The model under review builds one solid part; all positions refer to its coordinate system, in mm. Face numbers are marked on the shaded views. A direction names the side the tool comes from. Coordinates: 2 decimals unless noted, no trailing zeros. Loops run counter-clockwise (first coordinate to the right, second up) from the corner with the lowest first, then second, coordinate; pieces in that order, holes last. Notation, with made-up numbers: M 10.25,39.25 L 37.25,39.25 A19 cw 37.25,61.25 Z; hole C 35.25,-1.75 d10. An arc over 180 degrees is marked long. One line per item, written item: value.
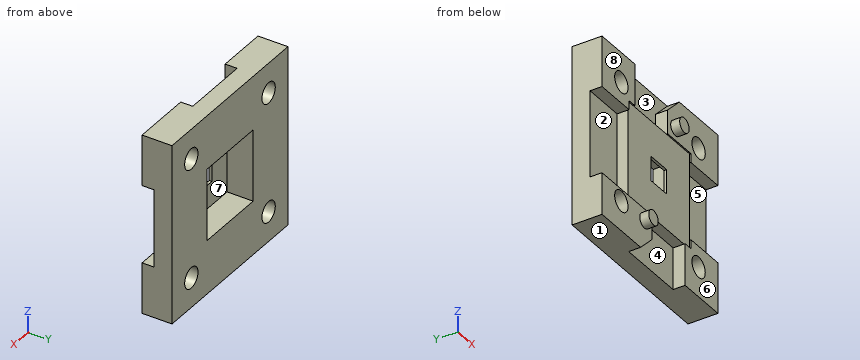
```python
from build123d import *

# Parameters (mm, degrees)
SKETCH_W        = 30
SKETCH_H        = 30
PAD_DEPTH       = 5
SKETCH001_W     = 7
SKETCH001_H     = 23
SKETCH001_W_2   = 23
SKETCH001_H_2   = 7
SKETCH001_H_3   = 16
SKETCH001_W_3   = 30
POCKET_DEPTH    = 2
SKETCH002_W     = 13
SKETCH002_H     = 7
PAD001_DEPTH    = 2
SKETCH003_R     = 1.725
POCKET001_DEPTH = 5.001
SKETCH004_R     = 1.225
PAD002_DEPTH    = 1.5
SKETCH005_W     = 7
SKETCH005_H     = 2
PAD003_DEPTH    = 1.5
SKETCH006_W     = 4.1
SKETCH006_H     = 4.1
POCKET002_DEPTH = 5
PAD004_DEPTH    = 2
SKETCH008_R     = 1.725
POCKET003_DEPTH = 5.001
PAD005_DEPTH    = 2
SKETCH010_R     = 1.725
POCKET004_DEPTH = 5.001
POCKET005_DEPTH = 2
SKETCH012_W     = 13
SKETCH012_H     = 7
PAD006_DEPTH    = 2
SKETCH013_R     = 1.725
POCKET006_DEPTH = 5.001
SKETCH014_R     = 1.225
PAD007_DEPTH    = 1.5
POCKET007_DEPTH = 2
SKETCH016_W     = 12
SKETCH016_H     = 12
POCKET008_DEPTH = 4.35
SKETCH017_W     = 16
SKETCH017_H     = 16
POCKET009_DEPTH = 0.2


with BuildPart() as part:
    # Sketch → Pad (new body)
    with BuildSketch(Plane.XZ):
        Rectangle(SKETCH_W, SKETCH_H)
    extrude(amount=-PAD_DEPTH)

    # Sketch001 (on Face5 of Pad) → Pocket (cut)
    with BuildSketch(Plane.XZ):
        with Locations((-11.5, 3.5)):
            Rectangle(SKETCH001_W, SKETCH001_H)
        with Locations((3.5, 11.5)):
            Rectangle(SKETCH001_W_2, SKETCH001_H_2)
        with Locations((11.5, 0)):
            Rectangle(SKETCH001_W, SKETCH001_H_3)
        with Locations((0, -11.5)):
            Rectangle(SKETCH001_W_3, SKETCH001_H_2)
    extrude(amount=-POCKET_DEPTH, mode=Mode.SUBTRACT)

    # Sketch002 (on Face2 of Pocket) → Pad001 (join)
    with BuildSketch(Plane.XZ.offset(-2)):
        with Locations((8.5, 11.5)):
            Rectangle(SKETCH002_W, SKETCH002_H)
    extrude(amount=PAD001_DEPTH)

    # Sketch003 (on Face15 of Pad001) → Pocket001 (cut, through all)
    with BuildSketch(Plane.XZ):
        with Locations((10, 10)):
            Circle(SKETCH003_R)
    extrude(amount=-POCKET001_DEPTH, mode=Mode.SUBTRACT)

    # Sketch004 (on Face15 of Pocket001) → Pad002 (join)
    with BuildSketch(Plane.XZ):
        with Locations((4, 10)):
            Circle(SKETCH004_R)
    extrude(amount=PAD002_DEPTH)

    # Sketch005 (on Face7 of Pad002) → Pad003 (join)
    with BuildSketch(Plane(origin=(0, 0, 8), x_dir=(1, 0, 0), z_dir=(0, 0, -1))):
        with Locations((11.5, -1)):
            Rectangle(SKETCH005_W, SKETCH005_H)
    extrude(amount=PAD003_DEPTH)

    # Sketch006 (on Face5 of Pad003) → Pocket002 (cut)
    with BuildSketch(Plane(origin=(0, 5, 0), x_dir=(1, 0, 0), z_dir=(0, 1, 0))):
        Rectangle(SKETCH006_W, SKETCH006_H)
    extrude(amount=-POCKET002_DEPTH, mode=Mode.SUBTRACT)

    # Sketch007 (on Face2 of Pocket002) → Pad004 (join)
    with BuildSketch(Plane.XZ.offset(-2)):
        Polygon((6.5, -15), (15, -15), (15, -6.5), (8, -6.5), (8, -8), (6.5, -8), align=None)
    extrude(amount=PAD004_DEPTH)

    # Sketch008 (on Face24 of Pad004) → Pocket003 (cut, through all)
    with BuildSketch(Plane.XZ):
        with Locations((10, -10)):
            Circle(SKETCH008_R)
    extrude(amount=-POCKET003_DEPTH, mode=Mode.SUBTRACT)

    # Sketch009 (on Face2 of Pocket003) → Pad005 (join)
    with BuildSketch(Plane.XZ.offset(-2)):
        Polygon((-15, 15), (-6.5, 15), (-6.5, 8), (-8, 8), (-8, 6.5), (-15, 6.5), align=None)
    extrude(amount=PAD005_DEPTH)

    # Sketch010 (on Face10 of Pad005) → Pocket004 (cut, through all)
    with BuildSketch(Plane.XZ):
        with Locations((-10, 10)):
            Circle(SKETCH010_R)
    extrude(amount=-POCKET004_DEPTH, mode=Mode.SUBTRACT)

    # Sketch011 (on Face14 of Pocket004) → Pocket005 (cut)
    with BuildSketch(Plane.XZ):
        Polygon((2, 15), (2, 12), (5, 15), align=None)
    extrude(amount=-POCKET005_DEPTH, mode=Mode.SUBTRACT)

    # Sketch012 (on Face28 of Pocket005) → Pad006 (join)
    with BuildSketch(Plane.XZ.offset(-2)):
        with Locations((-8.5, -11.5)):
            Rectangle(SKETCH012_W, SKETCH012_H)
    extrude(amount=PAD006_DEPTH)

    # Sketch013 (on Face42 of Pad006) → Pocket006 (cut, through all)
    with BuildSketch(Plane.XZ):
        with Locations((-10, -10)):
            Circle(SKETCH013_R)
    extrude(amount=-POCKET006_DEPTH, mode=Mode.SUBTRACT)

    # Sketch014 (on Face42 of Pocket006) → Pad007 (join)
    with BuildSketch(Plane.XZ):
        with Locations((-4, -10)):
            Circle(SKETCH014_R)
    extrude(amount=PAD007_DEPTH)

    # Sketch015 (on Face42 of Pad007) → Pocket007 (cut)
    with BuildSketch(Plane.XZ):
        Polygon((-2, -15), (-2, -12), (-5, -15), align=None)
    extrude(amount=-POCKET007_DEPTH, mode=Mode.SUBTRACT)

    # Sketch016 (on Face7 of Pocket007) → Pocket008 (cut)
    with BuildSketch(Plane(origin=(0, 5, 0), x_dir=(1, 0, 0), z_dir=(0, 1, 0))):
        Rectangle(SKETCH016_W, SKETCH016_H)
    extrude(amount=-POCKET008_DEPTH, mode=Mode.SUBTRACT)

    # Sketch017 (on Face32 of Pocket008) → Pocket009 (cut)
    with BuildSketch(Plane.XZ):
        Rectangle(SKETCH017_W, SKETCH017_H)
    extrude(amount=-POCKET009_DEPTH, mode=Mode.SUBTRACT)


solid = part.part
```
(1) Insertion check: pin 1 Ø13 at (x, z) = (2.5, -1.5) entering from -Y; pin 2 Ø10 at (x, z) = (-2.5, -10.5) entering from -Y; pin 3 Ø2 at (x, z) = (-1.5, -2) entering from +Y; pin 4 Ø0.5 at (y, z) = (0.5, -0.5) entering from +X. Each pin has a flat end and moves straight along its axis. Give the tip position at first contact, or say it passes through.
Checks:
pin 1: y = 0.2
pin 2: y = -1.5
pin 3: y = 0.65
pin 4: x = 8
(2) Add section D-D on z = -10. State the section outline as (x, y) points (3 decimals), then the cut area to 3 significant figures.
Checks:
outline: M -15,0 L -11.725,0 L -11.725,5 L -15,5 Z; M -8.275,0 L -5.225,0 L -5.225,-1.5 L -2.775,-1.5 L -2.775,0 L -2,0 L -2,2 L 6.5,2 L 6.5,0 L 8.275,0 L 8.275,5 L -8.275,5 Z; M 11.725,0 L 15,0 L 15,5 L 11.725,5 Z
area: 102 mm^2
(3) To check wall thickness, follow L1, parallel to Z at x = 10, y = 3.3 (3 decimals); L2, parallel to Z at x = 0.5, y = 2.25. State the ranges of each line that lie inside material, in increasing order. Write a range as [from, to].
Checks:
L1: [-15, -11.725], [-8.275, 8.275], [11.725, 15]
L2: [-15, -6], [6, 15]
(4) Add section C-C on y = 2.5. State the section outline as (x, z) points (3 decimals), then the cut area to 3 significant figures.
Checks:
outline: M -15,-15 L 15,-15 L 15,15 L -15,15 Z; hole C -10,-10 d3.45; hole C -10,10 d3.45; hole M -6,-6 L 6,-6 L 6,6 L -6,6 Z; hole C 10,-10 d3.45; hole C 10,10 d3.45
area: 719 mm^2
(5) Tool access review of the marked faces 4, 5, 6, 7 and 8: name each direction out of +Z, -Z, +X, -X, +Y, -Y from which nothing blocks a thin tool from reaching the whole face with its end or side.
Checks:
face 4: -Z, -Y
face 5: +X, -Y
face 6: +Z, -Z, +X, -Y
face 7: +Y
face 8: +Z, -Z, -X, -Y
(6) Add section B-B on z = -0.25. State the section outline as (x, y) points.
Checks:
outline: M -15,2 L -8,2 L -8,0.2 L -2.05,0.2 L -2.05,0.65 L -6,0.65 L -6,5 L -15,5 Z; M 2.05,0.2 L 8,0.2 L 8,2 L 15,2 L 15,5 L 6,5 L 6,0.65 L 2.05,0.65 Z
(7) Draft analysis for pull direction Z (two halves, no side actions). For the marked faces 1, 2 and 3, state which applies: pulls with the +Z half, pulls with the -Z half, needs draft (parallel to the pull), parting line crosses it, or undercut.
Checks:
face 1: pulls with the -Z half
face 2: undercut
face 3: needs draft
(8) Add section A-A on x = -10. State the section outline as (y, z) points (3 decimals), then the cut area to 3 significant figures.
Checks:
outline: M 0,-15 L 5,-15 L 5,-11.725 L 0,-11.725 Z; M 0,-8.275 L 5,-8.275 L 5,8.275 L 0,8.275 L 0,6.5 L 2,6.5 L 2,-8 L 0,-8 Z; M 0,11.725 L 5,11.725 L 5,15 L 0,15 Z
area: 86.5 mm^2
